from build123d import *

# Parameters (mm, degrees)
F0_W     = 50.8
F0_H     = 50.8
F1_DEPTH = 50.8
F2_W     = 43.208381
F2_H     = 44.698323
F3_DEPTH = 44.45
F4_R     = 10.414
F5_DEPTH = 50.801


with BuildPart() as f1:
    # F0 (on Top) → F1 (new body)
    with BuildSketch(Plane.XY):
        with Locations((0.893969, 10.03982)):
            Rectangle(F0_W, F0_H)
    extrude(amount=F1_DEPTH)

    # F2 (on face) → F3 (cut)
    with BuildSketch(Plane.XY.offset(50.8)):
        with Locations((0.446981, 9.982625)):
            Rectangle(F2_W, F2_H)
    extrude(amount=-F3_DEPTH, mode=Mode.SUBTRACT)

    # F4 (on face) → F5 (cut, through all)
    with BuildSketch(Plane(origin=(0, 0, 0), x_dir=(1, 0, 0), z_dir=(0, 0, -1))):
        with Locations((0, -10.386877)):
            Circle(F4_R)
    extrude(amount=-F5_DEPTH, mode=Mode.SUBTRACT)


solid = f1.part
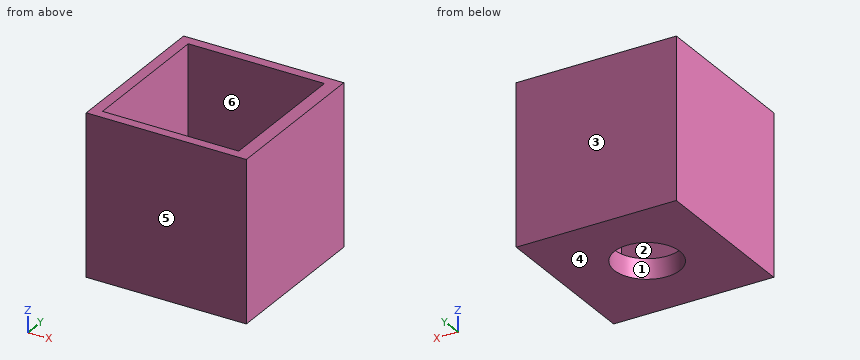
Model file for the job. Use its own axes, mm. Face numbers are marked on the shaded views. A direction names the side the tool comes from. Give positions to 0.01 mm unless a question says otherwise; leave off trailing zeros. Order: outer loops, then holes, each group sorted by start corner. A loop starts at its lowest first (then second) coordinate and runs counter-clockwise, first axis right, second up. Notation, with made-up numbers: (77.25, -14) -> (109.25, -14) arc R22 cw to (109.25, 0) -> close; hole circle Ø3 at (-27, 84.25). An arc over 180 degrees is marked (long way). Use CSV: the item, a comma, the result in double quotes.
1. 3-axis set-ups, long thin cutter, end or side, ignore diameter. For the marked faces 1 and 2: which of +Z, -Z, +X, -X, +Y, -Y reach the whole face in a straight line?
Outcome:
face 1,"+Z, -Z"
face 2,"+Z"
2. Band-saw the part on A-A, the plane x = 0. Give the cut face in (y, z), then the cut area to 3 significant figures.
Outcome:
outline,"(-15.36, 0) -> (-0.03, 0) -> (-0.03, 6.35) -> (-12.37, 6.35) -> (-12.37, 50.8) -> (-15.36, 50.8) -> close; (20.8, 0) -> (35.44, 0) -> (35.44, 50.8) -> (32.33, 50.8) -> (32.33, 6.35) -> (20.8, 6.35) -> close"
area,"462 mm²"
3. Band-saw the part on C-C, the plane y = 13.5. Give the cut face in (x, z), then the cut area to 3 significant figures.
Outcome:
outline,"(-24.51, 0) -> (-9.94, 0) -> (-9.94, 6.35) -> (-21.16, 6.35) -> (-21.16, 50.8) -> (-24.51, 50.8) -> close; (9.94, 0) -> (26.29, 0) -> (26.29, 50.8) -> (22.05, 50.8) -> (22.05, 6.35) -> (9.94, 6.35) -> close"
area,"534 mm²"
4. Drop a flat-ended pin along its axis: pin 1 (13 mm diameter, centred on x = 2.5, y = 18, fed in from +Z). Give the stop position or say it passes through.
Outcome:
pin 1,"z = 6.35"
5. Band-saw the part on B-B, the plane z = 31. Give the cut face in (x, y).
Outcome:
outline,"(-24.51, -15.36) -> (26.29, -15.36) -> (26.29, 35.44) -> (-24.51, 35.44) -> close; hole (-21.16, -12.37) -> (22.05, -12.37) -> (22.05, 32.33) -> (-21.16, 32.33) -> close"
6. Mould opens along Y. For the marked faces 3, 4, 5 and 6 say: +Y half, -Y half, draft (parallel to the pull), parting line (faces both ways), or undercut.
Outcome:
face 3,"+Y half"
face 4,"draft"
face 5,"-Y half"
face 6,"undercut"
7. Band-saw the part on D-D, the plane x = -14. Give the cut face in (y, z).
Outcome:
outline,"(-15.36, 0) -> (35.44, 0) -> (35.44, 50.8) -> (32.33, 50.8) -> (32.33, 6.35) -> (-12.37, 6.35) -> (-12.37, 50.8) -> (-15.36, 50.8) -> close"
8. Drill centre lines: line 1 along Y through (x, z) = (-11.5, 42); line 2 along X through (y, z) = (28, 15); line 3 along Z through (x, y) = (17.5, 8.5). Where is each one in solid material? Low to high. Write a range as from..to.
Outcome:
line 1,"-15.36..-12.37, 32.33..35.44"
line 2,"-24.51..-21.16, 22.05..26.29"
line 3,"0..6.35"
